```python
from build123d import *

# Parameters (mm, degrees)
SKETCH_1_R      = 35
SKETCH_1_R_2    = 30.85
EXTRUDE_1_DEPTH = 14
SKETCH_1_3_R    = 2.5
EXTRUDE_2_DEPTH = 6
SKETCH_1_4_R    = 2.5
EXTRUDE_3_DEPTH = 6


with BuildPart() as part:
    # Sketch 1 → Extrude 1 (new body)
    with BuildSketch(Plane(origin=(0, 0, 0), x_dir=(1, 0, 0), z_dir=(0, 1, 0))):
        with Locations(Location((0, 0, 0), (0, 0, 270))):
            Circle(SKETCH_1_R)
        with Locations(Location((0, 0, 0), (0, 0, 270))):
            Circle(SKETCH_1_R_2, mode=Mode.SUBTRACT)
    extrude(amount=EXTRUDE_1_DEPTH)

    # Sketch 1_3 → Extrude 2 (add)
    with BuildSketch(Plane(origin=(0, 0, 0), x_dir=(1, 0, 0), z_dir=(0, 1, 0))):
        with BuildLine():
            Line((50, -5), (34.641016151, -5))
            ThreePointArc((34.641016151, -5), (32.557544726, -12.845477081), (28.722813233, -20))
            Line((28.722813233, -20), (50, -20))
            Line((50, -20), (50, -5))
        make_face()
        with Locations(Location((42.290199458, -10, 0), (0, 0, 270))):
            Circle(SKETCH_1_3_R, mode=Mode.SUBTRACT)
    extrude(amount=EXTRUDE_2_DEPTH)

    # Sketch 1_4 → Extrude 3 (add)
    with BuildSketch(Plane(origin=(0, 0, 0), x_dir=(1, 0, 0), z_dir=(0, 1, 0))):
        with BuildLine():
            ThreePointArc((-28.722813233, -20), (-32.557544726, -12.845477081), (-34.641016151, -5))
            Line((-34.641016151, -5), (-50, -5))
            Line((-50, -5), (-50, -20))
            Line((-50, -20), (-28.722813233, -20))
        make_face()
        with Locations(Location((-42.290199458, -10, 0), (0, 0, 270))):
            Circle(SKETCH_1_4_R, mode=Mode.SUBTRACT)
    extrude(amount=EXTRUDE_3_DEPTH)


solid = part.part
```
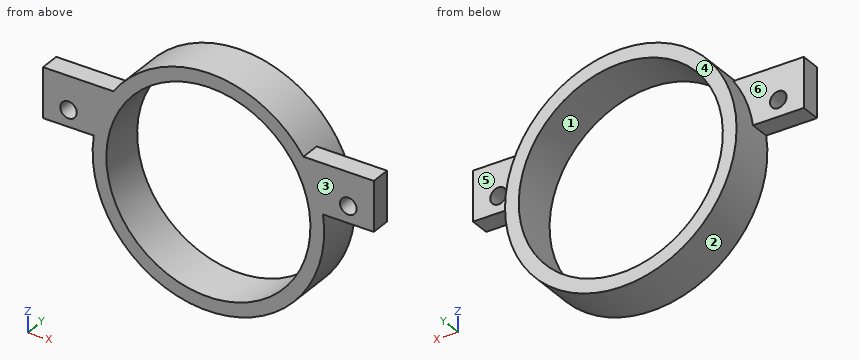
The model under review builds one solid part; all positions refer to its coordinate system, in mm. Face numbers are marked on the shaded views. A direction names the side the tool comes from. Round coordinates to 2 decimals unless told otherwise and drop trailing zeros. Loops run counter-clockwise (first coordinate to the right, second up) from the corner with the lowest first, then second, coordinate; pieces in that order, holes last. Notation, with made-up numbers: (38.5, -10) -> (63.5, -10) arc R19 cw to (63.5, 3) -> close; hole circle Ø1 at (-29.5, 14.25). An arc over 180 degrees is marked (long way). Answer as a JSON object with one key per item and string values. Group by question number.
1) We need section A-A on x = 0. Write out the cut boundary in (y, z), then the cut area to 3 significant figures.
2) We need section B-B on z = 0. Write out the cut boundary in (x, y).
3) For line 1 (X direction, y = 1.5, z = 10); line 2 (X direction, y = 9, z = 0); line 3 (X direction, y = 5, z = -24.5) (3 decimals), list the stretches that pass through material, from the lowest coordinate up. Write a range as [from, to].
4) We need section D-D on z = 11.5. Write out the cut boundary in (x, y), then the cut area to 3 significant figures.
5) For pin 1 Ø3 at (y, z) = (10.5, -4.5) entering from +X; pin 2 Ø7.5 at (x, z) = (-36, 9.5) entering from +Y; pin 3 Ø6.5 at (x, y) = (39, 2) entering from -Z; pin 4 Ø6.5 at (x, z) = (-42.29, 10) entering from +Y, all flat-tipped, find the tip position at first contact; note any pin that passes through.
6) Mouldability with a two-part tool opening along X and no side actions: class the marked faces 1, 2 and 3 as released by +X, released by -X, zero draft, split by the parting line, or undercut.
7) For the marked faces 4, 5 and 6, list the 3-axis set-ups (+Z, -Z, +X, -X, +Y, -Y) from which the entire face can be reached by the end or side of a thin tool; tool diameter is ignored.
8) We need section C-C on y = 13. Write out the cut boundary in (x, z).
Result set:
{
 "1": {"outline": "(0, -35) -> (14, -35) -> (14, -30.85) -> (0, -30.85) -> close; (0, 30.85) -> (14, 30.85) -> (14, 35) -> (0, 35) -> close", "area": "116 mm²"},
 "2": {"outline": "(-35, 0) -> (-30.85, 0) -> (-30.85, 14) -> (-35, 14) -> close; (30.85, 0) -> (35, 0) -> (35, 14) -> (30.85, 14) -> close"},
 "3": {"line 1": "[-50, -44.79], [-39.79, -29.18], [29.18, 39.79], [44.79, 50]", "line 2": "[-35, -30.85], [30.85, 35]", "line 3": "[-24.995, -18.748], [18.748, 24.995]"},
 "4": {"outline": "(-50, 0) -> (-44.29, 0) -> (-44.29, 6) -> (-50, 6) -> close; (-40.29, 0) -> (-28.63, 0) -> (-28.63, 14) -> (-33.06, 14) -> (-33.06, 6) -> (-40.29, 6) -> close; (28.63, 0) -> (40.29, 0) -> (40.29, 6) -> (33.06, 6) -> (33.06, 14) -> (28.63, 14) -> close; (44.29, 0) -> (50, 0) -> (50, 6) -> (44.29, 6) -> close", "area": "279 mm²"},
 "5": {"pin 1": "x = 34.87", "pin 2": "y = 14", "pin 3": "z = 5", "pin 4": "y = 6"},
 "6": {"face 1": "undercut", "face 2": "split by the parting line", "face 3": "zero draft"},
 "7": {"face 4": "+Z, -Z, +X, -X, +Y", "face 5": "+Z, +X, +Y", "face 6": "+Z, -X, +Y"},
 "8": {"outline": "circle Ø70 at (0, 0); hole circle Ø61.7 at (0, 0)"}
}
